```python
from build123d import *

# Parameters (mm, degrees)
SKETCH1_R           = 11
BOSS_EXTRUDE1_DEPTH = 5
SKETCH2_R           = 4
CUT_EXTRUDE3_DEPTH  = 3
CIRPATTERN1_COUNT   = 8


with BuildPart() as part:
    # Sketch1 → Boss-Extrude1 (new body, symmetric)
    with BuildSketch(Plane.XY):
        Polygon((6.213203436, 15), (-6.213203436, 15), (-15, 6.213203436), (-15, -6.213203436), (-6.213203436, -15), (6.213203436, -15), (15, -6.213203436), (15, 6.213203436), align=None)
        Circle(SKETCH1_R, mode=Mode.SUBTRACT)
    extrude(amount=BOSS_EXTRUDE1_DEPTH, both=True)

    # Sketch2 → Cut-Extrude3 (cut)
    with BuildSketch(Plane(origin=(0, -15, 0), x_dir=(-1, 0, 0), z_dir=(0, -1, 0))):
        Circle(SKETCH2_R)
    cut_extrude3 = extrude(amount=-CUT_EXTRUDE3_DEPTH, mode=Mode.SUBTRACT)

    # CirPattern1: Cut-Extrude3 ×8 about axis
    cirpattern1_axis = Axis((0, 0, 0), (0, 0, 1))
    for i in range(1, CIRPATTERN1_COUNT):
        add(cut_extrude3.rotate(cirpattern1_axis, i * 360 / CIRPATTERN1_COUNT), mode=Mode.SUBTRACT)


solid = part.part
```
Work out the finished part from the listing and answer in its coordinate system (mm). A direction names the side the tool comes from. Round coordinates to 2 decimals unless told otherwise and drop trailing zeros. Write each loop counter-clockwise with the first axis right and the second up, starting at its lowest first coordinate (ties: lowest second). Pieces come first, ordered by that corner, then holes.
1) A cutting plane is placed at C-C on x = -4.5. Determine the outline of the cut face in (y, z).
2) Flat-ended cylindrical pins translate along their axes: P1, Ø2.5, axis at x = -1, z = 1.5, coming from the +Y side; P2, Ø1, axis at x = -2.5, z = -2, coming from the -Y side; P3, Ø5, axis at y = 0, z = 0, coming from the -X side; P4, Ø13, axis at x = 0, y = 0, coming from the +Z side. Find the tip coordinate at first contact, or state that the pin passes through.
3) Consider probe 1 along Z at (x, y) = (0, -13.95); probe 2 along Y at (x, z) = (-2.75, 3.5); probe 3 along Y at (x, z) = (2.5, 2.25). Determine where each line is inside the solid, lowest interval first.
4) Determine the mould class of faces 1 (the face through (-8.45, -8.52, -0.06)), 2 (the face through (4.2, 15, 0.1)), 3 (the face through (-7, 10, 5)), 4 (the face through (13.521, 0.867, 3.905)) for opening direction Z: pulls with the +Z half, pulls with the -Z half, needs draft (parallel to the pull), parting line crosses it, or undercut.
5) Which of the six approach directions +Z, -Z, +X, -X, +Y, -Y give full straight-line access (tool end or side, diameter ignored) to faces 5 (the face through (-13.521, -0.867, 3.905)), 6 (the face through (0, 12, 0)), 7 (the face through (0.867, -13.521, 3.905))?
6) A cutting plane is placed at D-D on y = -7. Give the number of separate pieces and of enclosed holes in the cut face, and give its area (3 significant figures).
7) A cutting plane is placed at A-A on y = 0. Determine the outline of the cut face in (x, z).
Entries:
1. outline: (-15, -5) - (-10.04, -5) - (-10.04, 5) - (-15, 5) - close; (10.04, -5) - (15, -5) - (15, 5) - (10.04, 5) - close
2. P1: stops at y = 12
2. P2: stops at y = -12
2. P3: stops at x = -12
2. P4: passes through
3. probe 1: z = -5 to -4, 4 to 5
3. probe 2: y = -15 to -10.65, 10.65 to 15
3. probe 3: y = -12 to -10.71, 10.71 to 12
4. face 1: undercut
4. face 2: needs draft
4. face 3: pulls with the +Z half
4. face 4: undercut
5. face 5: -X
5. face 6: +Y
5. face 7: -Y
6. separate pieces: 2
6. enclosed holes: 2
6. area: 88.7 mm2
7. outline: (-15, -5) - (-11, -5) - (-11, 5) - (-15, 5) - (-15, 4) - (-12, 4) - (-12, -4) - (-15, -4) - close; (11, -5) - (15, -5) - (15, -4) - (12, -4) - (12, 4) - (15, 4) - (15, 5) - (11, 5) - close
